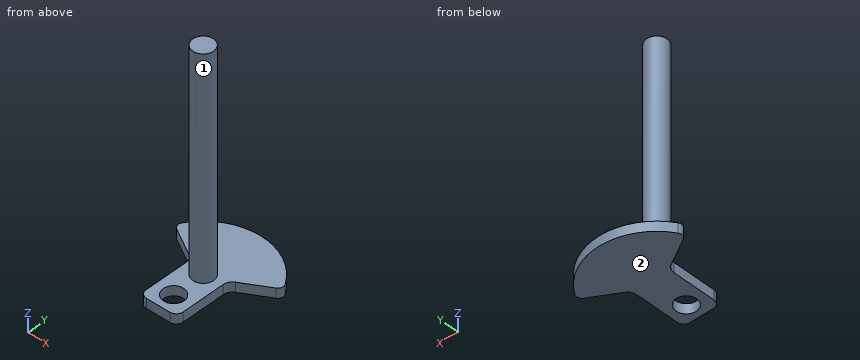
from build123d import *

# Parameters (mm, degrees)
SKETCH2_R           = 7.5
BOSS_EXTRUDE5_DEPTH = 7
SKETCH5_R           = 7.5
BOSS_EXTRUDE6_DEPTH = 165


with BuildPart() as part:
    # Sketch2 → Boss-Extrude5 (new body)
    with BuildSketch(Plane.XY):
        with BuildLine():
            Line((5, 0), (21.89510984, 0))
            ThreePointArc((21.89510984, 0), (25.430643746, 1.464466094), (26.89510984, 5))
            Line((26.89510984, 5), (26.89510984, 35.958548116))
            ThreePointArc((26.89510984, 35.958548116), (27.832932013, 39.458548116), (30.39510984, 42.020725942))
            Line((30.39510984, 42.020725942), (49.440130583, 53.016373795))
            ThreePointArc((49.440130583, 53.016373795), (51.323745621, 55.522595335), (50.821570497, 58.61726368))
            ThreePointArc((50.821570497, 58.61726368), (13.44755492, 79.210770001), (-23.926460657, 58.61726368))
            ThreePointArc((-23.926460657, 58.61726368), (-24.428635781, 55.522595335), (-22.545020743, 53.016373795))
            Line((-22.545020743, 53.016373795), (-3.5, 42.020725942))
            ThreePointArc((-3.5, 42.020725942), (-0.937822174, 39.458548116), (0, 35.958548116))
            Line((0, 35.958548116), (0, 5))
            ThreePointArc((0, 5), (1.464466094, 1.464466094), (5, 0))
        make_face()
        with Locations((13.44755492, 35)):
            Circle(SKETCH2_R, mode=Mode.SUBTRACT)
        with Locations((13.44755492, 12)):
            Circle(SKETCH2_R, mode=Mode.SUBTRACT)
    extrude(amount=BOSS_EXTRUDE5_DEPTH)

    # Sketch5 → Boss-Extrude6 (add)
    with BuildSketch(Plane(origin=(0, 0, 0), x_dir=(-1, 0, 0), z_dir=(0, 0, -1))):
        with Locations((-13.44755492, 35)):
            Circle(SKETCH5_R)
    extrude(amount=-BOSS_EXTRUDE6_DEPTH)


solid = part.part
Geometry check sheet. Reference: the model listing, model coordinates, mm. Face numbers are marked on the shaded views. A direction names the side the tool comes from. Round coordinates to 2 decimals unless told otherwise and drop trailing zeros. Loops run counter-clockwise (first coordinate to the right, second up) from the corner with the lowest first, then second, coordinate; pieces in that order, holes last.
Item 1: Cross-section at A-A on y = 12. Record the boundary of the cut face in (x, z).
Item 2: Cross-section at B-B on z = 116. Record the boundary of the cut face in (x, y), then the cut area to 3 significant figures.
Item 3: Gauge pin test, flat ends, axial feed: pin 1 (5.5 mm diameter, centred on y = 22, z = 5, fed in from -X); pin 2 (7.5 mm diameter, centred on y = 24, z = 2.5, fed in from +X); pin 3 (6 mm diameter, centred on y = 42, z = 64, fed in from -X). Record the tip position at first contact, or that the pin passes through.
Item 4: Cross-section at C-C on y = 50. Record the boundary of the cut face in (x, z).
Item 5: Access from +Z, -Z, +X, -X, +Y, -Y to the whole of each face (thin tool, end or side, straight path). Record for the marked faces 1 and 2.
Item 6: Cross-section at D-D on x = -16. Record the boundary of the cut face in (y, z).
Item 7: Thickness scan on line 1 (Z direction, x = -10, y = 50.5); line 2 (Y direction, x = 13, z = 150.5); line 3 (Y direction, x = 19, z = 151). Record the ranges inside material, lowest first.
Answer sheet:
1. outline: (0, 0) - (5.95, 0) - (5.95, 7) - (0, 7) - close; (20.95, 0) - (26.9, 0) - (26.9, 7) - (20.95, 7) - close
2. outline: circle Ø15 at (13.45, 35)
2. area: 177 mm2
3. pin 1: stops at x = 0
3. pin 2: stops at x = 26.9
3. pin 3: stops at x = 7.1
4. outline: (-17.32, 0) - (44.22, 0) - (44.22, 7) - (-17.32, 7) - close
5. face 1: +Z
5. face 2: -Z, +X, -X, +Y, -Y
6. outline: (49.24, 0) - (67.98, 0) - (67.98, 7) - (49.24, 7) - close
7. line 1: z = 0 to 7
7. line 2: y = 27.51 to 42.49
7. line 3: y = 29.96 to 40.04
